CAD build for the part. Positions are in the model's coordinates, mm. Face numbers are marked on the shaded views. Coordinates: 2 decimals unless noted, no trailing zeros. Use one line per item in the form item = value.
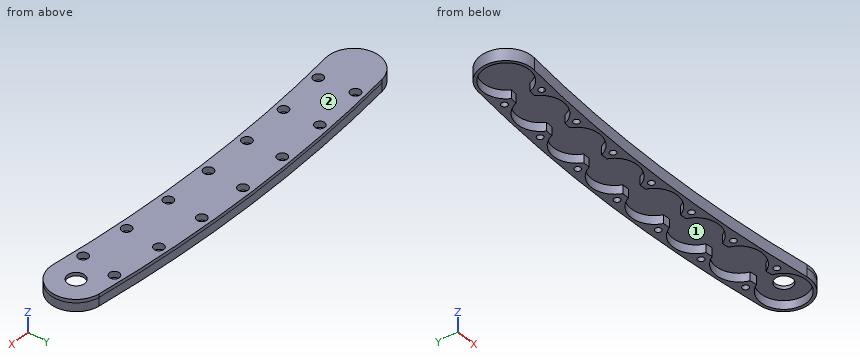
```python
from build123d import *

# Parameters (mm, degrees)
SKETCH1_R           = 13.3
BOSS_EXTRUDE1_DEPTH = 5
BOSS_EXTRUDE2_DEPTH = 2
CUT_EXTRUDE1_DEPTH  = 5
SKETCH4_R           = 5
CUT_EXTRUDE2_DEPTH  = 5
SKETCH5_R           = 1.775
CUT_EXTRUDE3_DEPTH  = 7
SKETCH6_R           = 2.875
CUT_EXTRUDE4_DEPTH  = 3.6


with BuildPart() as part:
    # Sketch1 → Boss-Extrude1 (new body)
    with BuildSketch(Plane.XY):
        with BuildLine():
            ThreePointArc((-97.97591629, 3.871645852), (-3.59e-07, 10), (97.975915577, 3.871645942))
            ThreePointArc((97.975915577, 3.871645942), (114.728175723, 16.885553085), (101.714268612, 33.637813256))
            ThreePointArc((101.714268612, 33.637813256), (2.3e-07, 40), (-101.714268155, 33.637813313))
            ThreePointArc((-101.714268155, 33.637813313), (-114.728175796, 16.88555367), (-97.97591629, 3.871645852))
        make_face()
        with Locations((-71.408926643, 21.811606454)):
            Circle(SKETCH1_R, mode=Mode.SUBTRACT)
        with BuildLine():
            ThreePointArc((84.645708431, 20.516381409), (70.223605302, 8.564530802), (58.152469631, 22.886942442))
            ThreePointArc((58.152469631, 22.886942442), (72.594247984, 35.058682105), (84.645708431, 20.516381409))
        make_face(mode=Mode.SUBTRACT)
        with Locations((99.845092065, 18.754729603)):
            Circle(SKETCH1_R, mode=Mode.SUBTRACT)
        with Locations((-42.881780686, 23.851690653)):
            Circle(SKETCH1_R, mode=Mode.SUBTRACT)
        with Locations((-14.3, 24.872382973)):
            Circle(SKETCH1_R, mode=Mode.SUBTRACT)
        with BuildLine():
            ThreePointArc((1.000606293, 24.999375218), (14.537366615, 38.17026465), (27.595453643, 24.524658339))
            ThreePointArc((27.595453643, 24.524658339), (14.062633385, 11.574501296), (1.000606293, 24.999375218))
        make_face(mode=Mode.SUBTRACT)
        with BuildLine():
            ThreePointArc((29.595391379, 24.453237978), (43.593578107, 37.132629792), (56.156354822, 23.029692169))
            ThreePointArc((56.156354822, 23.029692169), (42.169983266, 10.570751513), (29.595391379, 24.453237978))
        make_face(mode=Mode.SUBTRACT)
        with Locations((-99.845092065, 18.754729603)):
            Circle(SKETCH1_R, mode=Mode.SUBTRACT)
    extrude(amount=BOSS_EXTRUDE1_DEPTH)

    # Sketch2 → Boss-Extrude2 (add)
    with BuildSketch(Plane.XY.offset(5)):
        with BuildLine():
            ThreePointArc((101.714266956, 33.637813464), (0, 40), (-101.714266956, 33.637813464))
            ThreePointArc((-101.714266956, 33.637813464), (-114.728175927, 16.885554712), (-97.975917175, 3.871645741))
            ThreePointArc((-97.975917175, 3.871645741), (0, 10), (97.975917175, 3.871645741))
            ThreePointArc((97.975917175, 3.871645741), (114.728175927, 16.885554712), (101.714266956, 33.637813464))
        make_face()
    extrude(amount=BOSS_EXTRUDE2_DEPTH)

    # Sketch3 → Cut-Extrude1 (cut)
    with BuildSketch(Plane(origin=(0, 0, 0), x_dir=(-1, 0, 0), z_dir=(0, 0, -1))):
        with BuildLine():
            ThreePointArc((-87.020494046, 15.230572166), (-85.106230518, 15.438696412), (-83.191469288, 15.642190855))
            ThreePointArc((-83.191469288, 15.642190855), (-84.646494513, 20.524440227), (-84.159292066, 25.595543767))
            ThreePointArc((-84.159292066, 25.595543767), (-86.175068578, 25.381411595), (-88.190300336, 25.162211928))
            ThreePointArc((-88.190300336, 25.162211928), (-86.962958508, 22.062392675), (-86.545092065, 18.754729603))
            ThreePointArc((-86.545092065, 18.754729603), (-86.664478391, 16.976690466), (-87.020494046, 15.230572166))
        make_face()
        with BuildLine():
            ThreePointArc((-58.718270435, 17.832002829), (-56.797798717, 17.971677217), (-54.876994844, 18.106706988))
            ThreePointArc((-54.876994844, 18.106706988), (-56.156852796, 23.037773907), (-55.488980421, 28.088259411))
            ThreePointArc((-55.488980421, 28.088259411), (-57.51111487, 27.946203775), (-59.532885764, 27.799064431))
            ThreePointArc((-59.532885764, 27.799064431), (-58.469812615, 24.888833802), (-58.108926643, 21.811606454))
            ThreePointArc((-58.108926643, 21.811606454), (-58.262145144, 19.798614597), (-58.718270435, 17.832002829))
        make_face()
        with BuildLine():
            ThreePointArc((-30.341235174, 19.421711165), (-28.417002095, 19.492757738), (-26.492602834, 19.559150799))
            ThreePointArc((-26.492602834, 19.559150799), (-27.595662875, 24.532752701), (-26.747971493, 29.556185457))
            ThreePointArc((-26.747971493, 29.556185457), (-28.773887522, 29.486387348), (-30.799621658, 29.411495794))
            ThreePointArc((-30.799621658, 29.411495794), (-29.889807874, 26.697502042), (-29.581780686, 23.851690653))
            ThreePointArc((-29.581780686, 23.851690653), (-29.773019202, 21.604387303), (-30.341235174, 19.421711165))
        make_face()
        with BuildLine():
            ThreePointArc((-1.925542816, 19.997671761), (0, 20), (1.925542816, 19.997671761))
            ThreePointArc((1.925542816, 19.997671761), (1.000686071, 25.00747189), (2.027116435, 29.997451654))
            ThreePointArc((2.027116435, 29.997451654), (0, 30), (-2.027116435, 29.997451654))
            ThreePointArc((-2.027116435, 29.997451654), (-1.259306931, 27.485871884), (-1, 24.872382973))
            ThreePointArc((-1, 24.872382973), (-1.233434259, 22.391483998), (-1.925542816, 19.997671761))
        make_face()
        with BuildLine():
            ThreePointArc((26.492602834, 19.559150799), (28.417002095, 19.492757738), (30.341235174, 19.421711165))
            ThreePointArc((30.341235174, 19.421711165), (29.595760065, 24.461326646), (30.799621658, 29.411495794))
            ThreePointArc((30.799621658, 29.411495794), (28.773887522, 29.486387348), (26.747971493, 29.556185457))
            ThreePointArc((26.747971493, 29.556185457), (27.38525928, 27.252716893), (27.6, 24.872382973))
            ThreePointArc((27.6, 24.872382973), (27.320207711, 22.158678649), (26.492602834, 19.559150799))
        make_face()
        with BuildLine():
            ThreePointArc((54.876994844, 18.106706988), (56.797798717, 17.971677217), (58.718270435, 17.832002829))
            ThreePointArc((58.718270435, 17.832002829), (58.153126754, 22.895012799), (59.532885764, 27.799064431))
            ThreePointArc((59.532885764, 27.799064431), (57.51111487, 27.946203775), (55.488980421, 28.088259411))
            ThreePointArc((55.488980421, 28.088259411), (56.007437936, 25.998111339), (56.181780686, 23.851690653))
            ThreePointArc((56.181780686, 23.851690653), (55.851482847, 20.906045418), (54.876994844, 18.106706988))
        make_face()
        with BuildLine():
            ThreePointArc((83.191469288, 15.642190855), (85.106230518, 15.438696412), (87.020494046, 15.230572166))
            ThreePointArc((87.020494046, 15.230572166), (86.636401831, 20.310525956), (88.190300336, 25.162211928))
            ThreePointArc((88.190300336, 25.162211928), (86.175068578, 25.381411595), (84.159292066, 25.595543767))
            ThreePointArc((84.159292066, 25.595543767), (84.570800752, 23.723430175), (84.708926643, 21.811606454))
            ThreePointArc((84.708926643, 21.811606454), (84.323991823, 18.634958627), (83.191469288, 15.642190855))
        make_face()
    extrude(amount=-CUT_EXTRUDE1_DEPTH, mode=Mode.SUBTRACT)

    # Sketch4 → Cut-Extrude2 (cut)
    with BuildSketch(Plane(origin=(0, 0, 5), x_dir=(-1, 0, 0), z_dir=(0, 0, -1))):
        with Locations((-99.845092065, 18.754729603)):
            Circle(SKETCH4_R)
    extrude(amount=-CUT_EXTRUDE2_DEPTH, mode=Mode.SUBTRACT)

    # Sketch5 → Cut-Extrude3 (cut)
    with BuildSketch(Plane(origin=(0, 0, 0), x_dir=(-1, 0, 0), z_dir=(0, 0, -1))):
        with BuildLine():
            ThreePointArc((86.346811488, 10.467338821), (84.665812962, 12.239847981), (82.806767857, 10.655077946))
            ThreePointArc((82.806767857, 10.655077946), (84.571811488, 10.467338821), (86.336429526, 10.275640673))
            ThreePointArc((86.336429526, 10.275640673), (86.344214097, 10.371349284), (86.346811488, 10.467338821))
        make_face()
        with BuildLine():
            ThreePointArc((86.336429526, 10.275640673), (84.571811488, 10.467338821), (82.806767857, 10.655077946))
            ThreePointArc((82.806767857, 10.655077946), (84.382092732, 8.702506876), (86.336429526, 10.275640673))
        make_face()
        with Locations(Location((86.709487608, 30.352769186, 0), (0, 0, 180))):
            Circle(SKETCH5_R)
        with Locations(Location((57.867772947, 32.933467054, 0), (0, 0, 180))):
            Circle(SKETCH5_R)
        with Locations(Location((56.44114064, 12.984413937, 0), (0, 0, 180))):
            Circle(SKETCH5_R)
        with Locations(Location((28.238559382, 14.495942932, 0), (0, 0, 180))):
            Circle(SKETCH5_R)
        with Locations(Location((28.952330235, 34.483202153, 0), (0, 0, 180))):
            Circle(SKETCH5_R)
        with Locations((0, 35)):
            Circle(SKETCH5_R)
        with Locations((0, 15)):
            Circle(SKETCH5_R)
        with Locations((-28.238559382, 14.495942932)):
            Circle(SKETCH5_R)
        with Locations((-28.952330235, 34.483202153)):
            Circle(SKETCH5_R)
        with Locations((-56.44114064, 12.984413937)):
            Circle(SKETCH5_R)
        with Locations((-57.867772947, 32.933467054)):
            Circle(SKETCH5_R)
        with Locations((-86.709487608, 30.352769186)):
            Circle(SKETCH5_R)
        with Locations((-84.571811488, 10.467338821)):
            Circle(SKETCH5_R)
    extrude(amount=-CUT_EXTRUDE3_DEPTH, mode=Mode.SUBTRACT)

    # Sketch6 → Cut-Extrude4 (cut)
    with BuildSketch(Plane.XY.offset(7)):
        with Locations((-86.709487608, 30.352769186)):
            Circle(SKETCH6_R)
        with Locations((-84.571811488, 10.467338821)):
            Circle(SKETCH6_R)
        with Locations((-57.867772947, 32.933467054)):
            Circle(SKETCH6_R)
        with Locations((-56.44114064, 12.984413937)):
            Circle(SKETCH6_R)
        with Locations((-28.952330235, 34.483202153)):
            Circle(SKETCH6_R)
        with Locations((-28.238559382, 14.495942932)):
            Circle(SKETCH6_R)
        with Locations((0, 35)):
            Circle(SKETCH6_R)
        with Locations((0, 15)):
            Circle(SKETCH6_R)
        with Locations((28.952330235, 34.483202153)):
            Circle(SKETCH6_R)
        with Locations((28.238559382, 14.495942932)):
            Circle(SKETCH6_R)
        with Locations((57.867772947, 32.933467054)):
            Circle(SKETCH6_R)
        with Locations((56.44114064, 12.984413937)):
            Circle(SKETCH6_R)
        with Locations((86.709487608, 30.352769186)):
            Circle(SKETCH6_R)
        with Locations((84.571811488, 10.467338821)):
            Circle(SKETCH6_R)
    extrude(amount=-CUT_EXTRUDE4_DEPTH, mode=Mode.SUBTRACT)


solid = part.part
```
Item 1: Cut at A-A, the plane z = 2. State how many separate pieces and enclosed holes the cut face has, plus the area to 3 significant figures.
Derived:
separate_pieces = 1
enclosed_holes = 15
area = 1,940 mm²
Item 2: Drill centre lines: line 1 (Y direction, x = 0, z = 6) (3 decimals); line 2 (X direction, y = 26.5, z = 0.5); line 3 (X direction, y = 29, z = 5.75). Where is each one in solid material? Low to high. Write a range as [from, to].
Derived:
line_1 = [10, 12.125], [17.875, 32.125], [37.875, 40]
line_2 = [-112.69, -110.66], [-89.03, -83.86], [83.86, 89.03], [110.66, 112.69]
line_3 = [-110.8, -89.25], [-84.17, 84.17], [89.25, 110.8]
Item 3: Two-plate mould, pull along Y, no slides. Class the marked faces 1 and 2: +Y half, -Y half, draft (parallel to the pull), parting line (faces both ways), or undercut.
Derived:
face_1 = undercut
face_2 = draft
Item 4: Drop flat-ended pins along their axis: pin 1 (8 mm diameter, centred on x = 44.5, y = 20.5, fed in from -Z); pin 2 (1 mm diameter, centred on x = -58, z = 1, fed in from -Y); pin 3 (4.5 mm diameter, centred on x = -86.71, y = 30.35, fed in from +Z); pin 4 (3 mm diameter, centred on x = -86.71, y = 30.35, fed in from +Z). Give the stop position or say it passes through.
Derived:
pin_1 = 5
pin_2 = 7.82
pin_3 = 3.4
pin_4 = through
